Autodesk Inventor part; units mm, degrees
ref_plane "YZ Plane" through (0, 0, 0) normal (1, 0, 0) x (0, 1, 0)
ref_plane "XZ Plane" through (0, 0, 0) normal (0, 1, 0) x (-1, 0, 0)
ref_plane "XY Plane" through (0, 0, 0) normal (0, 0, 1) x (1, 0, 0)
sketch "Sketch1" plane through (0, 0, 0) normal (0, 0, 1) x (1, 0, 0)
  arc A0 (-26.67, -12.5235) -> (26.67, -12.5235) centre (0, 0) ccw
  line L0 (-26.67, -12.5235) -> (-26.67, 21.7665)
  line L1 (-26.67, 21.7665) -> (-15.24, 21.7665)
  line L2 (-15.24, 21.7665) -> (-15.24, 14.1465)
  line L3 (-15.24, 14.1465) -> (15.24, 14.1465)
  line L4 (15.24, 14.1465) -> (15.24, 21.7665)
  line L5 (15.24, 21.7665) -> (26.67, 21.7665)
  line L6 (26.67, 21.7665) -> (26.67, -12.5235)
  line L7 (-17.018, 6.5265) -> (6.096, 6.5265)
  line L8 (6.096, 6.5265) -> (6.096, -6.1735)
  line L9 (6.096, -6.1735) -> (-17.018, -6.1735)
  line L10 (-17.018, -6.1735) -> (-17.018, 6.5265)
  line L11 (-5.588, -6.1735) -> (-2.794, -6.1735)
  line L12 (-2.794, -6.1735) -> (-2.794, -7.9515)
  line L13 (-2.794, -7.9515) -> (-5.588, -7.9515)
  line L14 (-5.588, -7.9515) -> (-5.588, -6.1735)
  line L15 (4.572, -6.1735) -> (7.366, -6.1735)
  line L16 (7.366, -6.1735) -> (7.366, -7.9515)
  line L17 (7.366, -7.9515) -> (4.572, -7.9515)
  line L18 (4.572, -7.9515) -> (4.572, -6.1735)
  line L19 (9.906, -7.9515) -> (11.938, -7.9515)
  line L20 (11.938, -7.9515) -> (11.938, -20.1435)
  line L21 (11.938, -20.1435) -> (9.906, -20.1435)
  line L22 (9.906, -20.1435) -> (9.906, -7.9515)
  line L23 (-5.588, -20.1435) -> (-2.794, -20.1435)
  line L24 (-2.794, -20.1435) -> (-2.794, -21.9215)
  line L25 (-2.794, -21.9215) -> (-5.588, -21.9215)
  line L26 (-5.588, -21.9215) -> (-5.588, -20.1435)
  line L27 (-8.382, -12.5235) -> (-6.604, -12.5235)
  line L28 (-6.604, -12.5235) -> (-6.604, -15.3175)
  line L29 (-6.604, -15.3175) -> (-8.382, -15.3175)
  line L30 (-8.382, -15.3175) -> (-8.382, -12.5235)
  line L31 (-13.97, -12.5235) -> (-12.192, -12.5235)
  line L32 (-12.192, -12.5235) -> (-12.192, -15.3175)
  line L33 (-12.192, -15.3175) -> (-13.97, -15.3175)
  line L34 (-13.97, -15.3175) -> (-13.97, -12.5235)
  line L35 (20.574, 1.1925) -> (22.352, 1.1925)
  line L36 (22.352, 1.1925) -> (22.352, -1.6015)
  line L37 (22.352, -1.6015) -> (20.574, -1.6015)
  line L38 (20.574, -1.6015) -> (20.574, 1.1925)
  line L39 (4.572, -20.1435) -> (7.366, -20.1435)
  line L40 (7.366, -20.1435) -> (7.366, -21.9215)
  line L41 (7.366, -21.9215) -> (4.572, -21.9215)
  line L42 (4.572, -21.9215) -> (4.572, -20.1435)
  circle A1 centre (-23.368, 18.4645) radius 1.524
  circle A2 centre (-23.368, 10.3365) radius 1.524
  circle A3 centre (-23.368, -11.5075) radius 1.524
  circle A4 centre (-19.304, 0.1765) radius 1.27
  circle A5 centre (8.382, 0.1765) radius 1.27
  circle A6 centre (23.368, 18.4645) radius 1.524
  circle A7 centre (23.368, 10.3365) radius 1.524
  circle A8 centre (23.368, -11.5075) radius 1.524
  dimension "d0" = 29.464
  dimension "d1" = 34.29
  dimension "d2" = 11.43
  dimension "d3" = 7.62
  dimension "d4" = 30.48
  dimension "d5" = 2.794
  dimension "d6" = 12.7
  dimension "d7" = 23.114
  dimension "d8" = 7.62
  dimension "d9" = 9.652
  dimension "d10" = 1.778
  dimension "d11" = 12.954
  dimension "d12" = 4.318
  dimension "d13" = 12.192
  dimension "d14" = 7.366
  dimension "d15" = 2.032
  dimension "d16" = 2.54
  dimension "d17" = 1.27
  dimension "d18" = 1.016
  dimension "d19" = 4.572
  dimension "d20" = 3.81
  dimension "d21" = 3.048
  dimension "d22" = 2.54
  dimension "d23" = 3.302
  dimension "d24" = 3.302
  dimension "d25" = 3.302
  dimension "d26" = 3.302
  dimension "d27" = 8.128
  dimension "d28" = 21.844
  dimension "d29" = 2.286
  dimension "d30" = 2.286
  dimension "d31" = 6.35
extrude "Extrusion1" add sketch "Sketch1" along normal blind 3.175
properties part number "PixyCamGimbal Body"
Read the model definition and answer for the solid it produces. Units are mm, in the model's axes. A direction names the side the tool comes from. Round coordinates to 2 decimals unless told otherwise and drop trailing zeros. Write each loop counter-clockwise with the first axis right and the second up, starting at its lowest first coordinate (ties: lowest second). Pieces come first, ordered by that corner, then holes. Notation, with made-up numbers: M -32.5,68 L 4.5,68 A29 cw 4.5,95 Z; hole C -37.75,-22 d11. An arc over 180 degrees is marked long. One line per item, written item: value.
Q1. Which of the six approach directions +Z, -Z, +X, -X, +Y, -Y give full straight-line access (tool end or side, diameter ignored) to faces 5 (the flat face through (1, -6.174, 2)), 6 (the flat face through (-26.67, 4, 2))?
Data:
face 5: +Z, -Z
face 6: +Z, -Z, -X, +Y, -Y
Q2. Find section C-C on z = 2. Count the separate pieces of the cut face and the enclosed holes in it, plus the area to 3 significant figures.
Data:
separate pieces: 1
enclosed holes: 15
area: 1,840 mm2
Q3. For a pull along Y with two mould halves and no side action, classify faces 1 (the flat face through (-17.018, 0, 2)), 2 (the cylindrical face through (0.47, -29.46, 1.57)), 3 (the flat face through (-6.604, -14, 2)), 4 (the flat face through (0, -9, 0)) as +Y half, -Y half, draft (parallel to the pull), parting line (faces both ways), or undercut.
Data:
face 1: undercut
face 2: -Y half
face 3: undercut
face 4: draft
Q4. Find section D-D on x = 14. Write down the section's boundary in (y, z) (1 decimal), plus the area to 3 significant figures.
Data:
outline: M -25.9,0 L 14.1,0 L 14.1,3.2 L -25.9,3.2 Z
area: 127 mm2
Q5. Flat-ended cylindrical pins translate along their axes: pin 1 Ø8 at (x, y) = (-3, 5.5) entering from +Z (3 decimals); pin 2 Ø0.5 at (x, z) = (-13.5, 2) entering from -Y; pin 3 Ø1.4 at (y, z) = (-21, 2.5) entering from +X (3 decimals); pin 4 Ø0.5 at (y, z) = (-21, 1.5) entering from -X. Find the tip coordinate at first contact, or state that the pin passes through.
Data:
pin 1: z = 3.175
pin 2: y = -26.32
pin 3: x = 21.355
pin 4: x = -20.92
Q6. Straight lines are drawn through the part: line 1 (Y direction, x = -23, z = 0.9); line 2 (X direction, y = -21.5, z = 3); line 3 (X direction, y = -3.5, z = 2.4). For each, find the intervals that lie inside material, in ascending order. Write a range as [from, to].
Data:
line 1: [-18.42, -12.99], [-10.03, 8.86], [11.82, 16.99], [19.94, 21.77]
line 2: [-20.15, -5.59], [-2.79, 4.57], [7.37, 20.15]
line 3: [-26.67, -17.02], [6.1, 26.67]
Q7. Find section B-B on y = -14. Write down the section's boundary in (x, z) (3 decimals).
Data:
outline: M -25.925,0 L -13.97,0 L -13.97,3.175 L -25.925,3.175 Z; M -12.192,0 L -8.382,0 L -8.382,3.175 L -12.192,3.175 Z; M -6.604,0 L 9.906,0 L 9.906,3.175 L -6.604,3.175 Z; M 11.938,0 L 25.925,0 L 25.925,3.175 L 11.938,3.175 Z
Q8. Find section A-A on y = -2.5. Write down the section's boundary in (x, z) (3 decimals).
Data:
outline: M -26.67,0 L -17.018,0 L -17.018,3.175 L -26.67,3.175 Z; M 6.096,0 L 26.67,0 L 26.67,3.175 L 6.096,3.175 Z
